Geometry: final body of the model. Coordinates: model frame, mm. A direction names the side the tool comes from. Round coordinates to 2 decimals unless told otherwise and drop trailing zeros. Write each loop counter-clockwise with the first axis right and the second up, starting at its lowest first coordinate (ties: lowest second). Pieces come first, ordered by that corner, then holes. Notation, with made-up numbers: M 77,-23.75 L 126,-23.75 A13 ccw 126,-11.75 Z; hole C -11,50 d3. An arc over 180 degrees is marked long. Use one line per item in the form item = value. Start each with the question number.
Item 1: Pull-direction query (Y, two-part tool) for faces 1 (the cylindrical face through (2.61, 21.76, -0.63)), 2 (the flat face through (5, -2, 0)), 3 (the flat face through (2.2, -3.3, 20)); classes: pulls with the +Y half, pulls with the -Y half, needs draft (parallel to the pull), parting line crosses it, or undercut.
Item 2: Section query A-A (y = 15.5). Return loops of the section in (x, z), and give its area (3 significant figures).
Item 3: Section query D-D (y = -3). Return loops of the section in (x, z).
Item 4: Ray query, probe 1 along Z at (x, y) = (-1.5, 15.5); probe 2 along Z at (x, y) = (-3.25, 17.5); probe 3 along Z at (x, y) = (-4.75, 0.5). Return the intervals inside material, ascending.
Item 5: Pin query (flat end, axial travel): pin 1 Ø10 at (x, y) = (0.5, 0.5) entering from +Z; pin 2 Ø9 at (x, y) = (0, 0) entering from -Z; pin 3 Ø1.5 at (x, z) = (-5.5, 23.5) entering from -Y. Return the tip coordinate at first contact, or that it passes through.
Item 6: Reachability of faces 4 (the cylindrical face through (3.233, -1.341, 17.465)), 5 (the flat face through (-5, 16, 17)), 6 (the cylindrical face through (-1.08, -4.88, 7.4)), 7 (the flat face through (2.6, 18.5, 36.2)), 8 (the flat face through (5, -2, 35)) from +Z, -Z, +X, -X, +Y, -Y: full face, straight path, thin tool, end or side. Return the list, or none.
Item 7: Section query B-B (z = 4). Return loops of the section in (x, y).
Item 8: Section query C-C (x = 0). Return loops of the section in (y, z), and give its area (3 significant figures).
from build123d import *

# Parameters (mm, degrees)
SKETCH1_R                = 5
BOSS_EXTRUDE1_DEPTH      = 15
SKETCH3_R                = 3.5
BOSS_EXTRUDE2_DEPTH      = 5
SKETCH4_R                = 5
BOSS_EXTRUDE3_DEPTH      = 15
BOSS_EXTRUDE4_DEPTH      = 5
BOSS_EXTRUDE4_DEPTH_BACK = 10
SKETCH7_R                = 2.45
CUT_EXTRUDE1_DEPTH       = 48.86961474
CUT_EXTRUDE2_DEPTH       = 50.663870332


with BuildPart() as part:
    # Sketch1 → Boss-Extrude1 (new body)
    with BuildSketch(Plane.XY):
        with BuildLine():
            Line((0, 12), (10, 12))
            Line((10, 12), (10, 0))
            ThreePointArc((10, 0), (-7.071067812, -7.071067812), (0, 10))
            Line((0, 10), (0, 12))
        make_face()
        Circle(SKETCH1_R, mode=Mode.SUBTRACT)
    extrude(amount=BOSS_EXTRUDE1_DEPTH)

    # Sketch3 → Boss-Extrude2 (add)
    with BuildSketch(Plane.XY.offset(15)):
        with BuildLine():
            Line((10, 0), (10, 12))
            Line((10, 12), (0, 12))
            Line((0, 12), (0, 10))
            ThreePointArc((0, 10), (-7.071067812, 7.071067812), (-10, 0))
            ThreePointArc((-10, 0), (0, -10), (10, 0))
        make_face()
        Circle(SKETCH3_R, mode=Mode.SUBTRACT)
    extrude(amount=BOSS_EXTRUDE2_DEPTH)

    # Sketch4 → Boss-Extrude3 (add)
    with BuildSketch(Plane.XY.offset(20)):
        with BuildLine():
            Line((0, 12), (10, 12))
            Line((10, 12), (10, 0))
            ThreePointArc((10, 0), (-7.071067812, -7.071067812), (0, 10))
            Line((0, 10), (0, 12))
        make_face()
        with Locations(Location((0, 0, 0), (0, 0, 180))):
            Circle(SKETCH4_R, mode=Mode.SUBTRACT)
    extrude(amount=BOSS_EXTRUDE3_DEPTH)

    # Sketch6 → Boss-Extrude4 (add, two sides: drawn at the far end of the back side and taken through both)
    with BuildSketch(Plane.ZY.offset(-BOSS_EXTRUDE4_DEPTH_BACK)):
        with BuildLine():
            Line((9.5, 22.5), (2.5, 22.5))
            ThreePointArc((2.5, 22.5), (-4.5, 15.5), (2.5, 8.5))
            Line((2.5, 8.5), (32.5, 8.5))
            ThreePointArc((32.5, 8.5), (39.5, 15.5), (32.5, 22.5))
            Line((32.5, 22.5), (25.5, 22.5))
            Line((25.5, 22.5), (9.5, 22.5))
        make_face()
    extrude(amount=BOSS_EXTRUDE4_DEPTH + BOSS_EXTRUDE4_DEPTH_BACK)

    # Sketch7 → Cut-Extrude1 (cut, through all)
    with BuildSketch(Plane.ZY.offset(5)):
        with Locations((2.5, 15.5)):
            Circle(SKETCH7_R)
        with Locations((32.5, 15.5)):
            Circle(SKETCH7_R)
    extrude(amount=-CUT_EXTRUDE1_DEPTH, mode=Mode.SUBTRACT)

    # Sketch8 → Cut-Extrude2 (cut, through all)
    with BuildSketch(Plane(origin=(10, 0, 0), x_dir=(0, 0, -1), z_dir=(1, 0, 0))):
        Polygon((-32.125, 16.149519053), (-32.875, 14.850480947), (-38.937177826, 18.350480947), (-38.187177826, 19.649519053), align=None)
        Polygon((-2.875, 16.149519053), (-2.125, 14.850480947), (3.937177826, 18.350480947), (3.187177826, 19.649519053), align=None)
    extrude(amount=-CUT_EXTRUDE2_DEPTH, mode=Mode.SUBTRACT)


solid = part.part
Working result:
q1.face_1 = pulls with the +Y half
q1.face_2 = needs draft
q1.face_3 = undercut
q2.outline = M -5,-4.5 L 10,-4.5 L 10,0.05 L -5,0.05 Z; M -5,4.95 L 10,4.95 L 10,30.05 L -5,30.05 Z; M -5,34.95 L 10,34.95 L 10,39.5 L -5,39.5 Z
q2.area = 513 mm²
q3.outline = M -9.54,0 L -4,0 L -4,15 L -1.8,15 L -1.8,20 L -4,20 L -4,35 L -9.54,35 Z; M 1.8,15 L 4,15 L 4,0 L 9.54,0 L 9.54,35 L 4,35 L 4,20 L 1.8,20 Z
q4.probe_1 = -4.5 to 0.05, 4.95 to 30.05, 34.95 to 39.5
q4.probe_2 = -4.21 to -2.46, 0.54 to 1.08, 3.92 to 31.08, 33.92 to 34.46, 37.46 to 39.21
q4.probe_3 = 15 to 20
q5.pin_1 = 35
q5.pin_2 = 15
q5.pin_3 = -8.8
q6.face_4 = +Z, -Z
q6.face_5 = +Z, -Z, -X, +Y
q6.face_6 = -Z
q6.face_7 = +X, -X
q6.face_8 = +Z, +X, -X, -Y
q7.outline = M -5,8.66 A10 ccw long 10,0 L 10,13.56 L -5,13.56 Z; M -5,17.44 L 10,17.44 L 10,22.5 L -5,22.5 Z; hole C 0,0 d10
q8.outline = M -10,0 L -5,0 L -5,15 L -3.5,15 L -3.5,20 L -5,20 L -5,35 L -10,35 Z; M 3.5,15 L 5,15 L 5,0 L 8.96,0 A7 ccw 18.33,-3.9 L 16.02,0.11 A2.45 cw long 17.32,0.86 L 19.63,-3.15 A7 ccw 22.5,2.5 L 22.5,32.5 A7 ccw 19.63,38.15 L 17.32,34.14 A2.45 cw long 16.02,34.89 L 18.33,38.9 A7 ccw 8.96,35 L 5,35 L 5,20 L 3.5,20 Z
q8.area = 836 mm²
